The listing builds one solid part. Answer for the finished solid, in the listing's coordinates (mm). Face numbers are marked on the shaded views. A direction names the side the tool comes from. Give positions to 0.01 mm unless a question says otherwise; leave off trailing zeros. Loops run counter-clockwise (first coordinate to the right, second up) from the corner with the lowest first, then second, coordinate; pieces in that order, holes last. Notation, with made-up numbers: (-6, 56.25) - (6, 56.25) arc R20 cw to (6, 94.25) - close; hole circle Ø11 at (16, 21). An arc over 180 degrees is marked (long way). Write item = value, one per line. Start each with the question number.
1) Consider probe 1 along Z at (x, y) = (43.5, 22); probe 2 along Y at (x, z) = (63, 7.25); probe 3 along Y at (x, z) = (34.5, 4.25). Determine where each line is inside the solid, lowest interval first.
2) The part is cut by section C-C on z = 10.25. State how many separate pieces and enclosed holes the cut face has, plus the area to 3 significant figures.
3) Which of the six approach directions +Z, -Z, +X, -X, +Y, -Y give full straight-line access (tool end or side, diameter ignored) to the marked faces 1, 2, 3 and 4?
4) The part is cut by section B-B on x = 48.5. Write down the section's boundary in (y, z).
5) The mould has two halves that part along X. Classify the marked faces 5, 6 and 7: +X half, -X half, draft (parallel to the pull), parting line (faces both ways), or undercut.
6) Flat-ended cylindrical pins translate along their axes: P1, Ø1.5, axis at x = 74, z = 9, coming from the +Y side; P2, Ø7.5, axis at y = 44.5, z = 5, coming from the +X side; P3, Ø4.5, axis at y = 41, z = 6.5, coming from the +X side. Find the tip coordinate at first contact, or state that the pin passes through.
from build123d import *

# Parameters (mm, degrees)
BOSS_EXTRUDE1_DEPTH = 7
SKETCH1_3_R         = 7.578000113984699
BOSS_EXTRUDE2_DEPTH = 14.5
FILLET1_R           = 2


with BuildPart() as part:
    # Sketch1 → Boss-Extrude1 (new body)
    with BuildSketch(Plane.XY):
        with BuildLine():
            Line((78.96827475522947, 42.187825253742076), (71.54074542683735, 53.865587102003296))
            add(Edge.make_bspline(
                [(68.3903409242589, 57.6204965379541), (68.60270993607134, 57.450222077167965), (69.77589066925935, 56.287697416771124), (70.76711290567236, 54.99803586851411), (71.54074542683735, 53.865587102003296)],
                knots=[0.22419046507503326, 0.22419046507503326, 0.22419046507503326, 0.22419046507503326, 0.35338295041403034, 1, 1, 1, 1], degree=3))
            add(Edge.make_bspline(
                [(67.16681294608784, 58.3330475317527), (67.53066578937491, 58.14815845494029), (67.96561960838265, 57.94613577996738), (68.34100319904479, 57.66005482607508), (68.3903409242589, 57.6204965379541)],
                knots=[0, 0, 0, 0, 0.19417637174294056, 0.22419046507503326, 0.22419046507503326, 0.22419046507503326, 0.22419046507503326], degree=3))
            Line((67.16681294608784, 58.3330475317527), (56.03811631838445, 62.90331689854259))
            Line((56.03811631838445, 62.90331689854259), (50.21233359803197, 48.7174203330503))
            Line((50.21233359803197, 48.7174203330503), (52.95464713088683, 47.643030748312306))
            ThreePointArc((52.95464713088681, 47.64303074831224), (57.760447877225054, 40.24223776631537), (52.30143900683574, 33.30922401118043))
            Line((52.30143900683574, 33.30922401118043), (20.622854324708115, 24.120186594388674))
            Line((20.622854324708115, 24.120186594388674), (20.62282110130341, 6.139939904360626))
            Line((20.62282110130341, 6.139939904360626), (20.62282110130341, 6.062388021954931))
            Line((20.62282110130341, 6.062388021954931), (83.96827475522947, 15.843555634253288))
            add(Edge.make_bspline(
                [(83.96827475522947, 15.843555634253288), (85.80036579939097, 15.861062531667944), (88.17372578299519, 16.28932128394429), (90.97579799916589, 17.070964386264627), (92.71201966041953, 17.824393939393527), (94.43214299682957, 19.052982353729515), (96.04268050119445, 20.454120961956406), (97.16419489006465, 21.752212782610812), (97.85208586964548, 22.923017737887626), (98.59154777476378, 23.895634779714683), (99.07674499256737, 25.078186890956406), (99.65372100416238, 26.703400446360803), (99.9224179321126, 28.680656555027426), (100.1456525457167, 30.848800013363814), (100.51886620718611, 32.862374788732254), (101.11013591134653, 34.64525635165334), (101.50715414680975, 36.22789720071845), (102.06593723414899, 37.400646367775394), (102.48628027717764, 38.406589288866975), (102.84842112165893, 39.429390424414976), (103.21090056683431, 39.99039765339784), (103.38837792674808, 40.31628873971178)],
                knots=[0, 0, 0, 0, 0.1578550410840074, 0.20703944686554082, 0.2510949501731389, 0.3205511449351055, 0.3885120157665865, 0.43536001171879174, 0.4678008080744776, 0.5056992154510483, 0.5402779798217185, 0.5775724755717133, 0.6545316786338135, 0.7114166705153907, 0.7661367857027547, 0.8308692773593267, 0.873613048584834, 0.90658473443976, 0.9427498705208139, 0.9678813230428206, 1, 1, 1, 1], degree=3))
            Line((103.38837792674808, 40.31628873971178), (103.5353457354515, 40.58470837115218))
            Line((103.5353457354515, 40.58470837115218), (98.46827475522947, 40.584708371152175))
            Line((98.46827475522947, 40.584708371152175), (98.46827475522947, 57.7986883791206))
            Line((98.46827475522947, 57.7986883791206), (88.96827475522947, 57.7986883791206))
            Line((88.96827475522947, 57.7986883791206), (88.96827475522946, 31.5935556342533))
            ThreePointArc((88.96827475522946, 31.5935556342533), (83.96827475522947, 26.593555634253313), (78.96827475522949, 31.593555634253303))
            Line((78.96827475522947, 31.593555634253303), (78.96827475522947, 42.187825253742076))
        make_face()
    extrude(amount=BOSS_EXTRUDE1_DEPTH)

    # Sketch1_3 → Boss-Extrude2 (add)
    with BuildSketch(Plane.XY):
        with BuildLine():
            Line((52.95464713088683, 47.643030748312306), (50.21233359803197, 48.7174203330503))
            Line((50.21233359803197, 48.7174203330503), (23.91329061275728, 59.02091682731907))
            Line((23.91329061275728, 59.02091682731907), (22.08936487086497, 54.365458215317176))
            Line((22.08936487086497, 54.365458215317176), (40.01978708427513, 47.34063824296787))
            Line((40.01978708427513, 47.34063824296787), (44.49575262392416, 45.58703468895018))
            ThreePointArc((44.49575262392417, 45.58703468895018), (48.4005247200828, 47.95082949329833), (52.95464713088681, 47.64303074831224))
        make_face()
        with Locations((50.19030425910602, 40.58721795212874)):
            Circle(SKETCH1_3_R)
        with BuildLine():
            ThreePointArc((43.63005434703988, 36.79390715299979), (42.648765078906784, 41.32969523869845), (44.49575262392417, 45.58703468895018))
            Line((44.49575262392416, 45.58703468895018), (40.01978708427513, 47.34063824296787))
            Line((40.01978708427513, 47.34063824296787), (40.019787084275116, 35.746673468318164))
            Line((40.01978708427511, 35.74667346831816), (43.63005434703988, 36.79390715299979))
        make_face()
        with BuildLine():
            Line((20.622854324708115, 24.120186594388674), (52.30143900683574, 33.30922401118043))
            ThreePointArc((52.30143900683574, 33.30922401118043), (47.364634323302816, 33.55574050130448), (43.63005434703988, 36.79390715299979))
            Line((43.63005434703988, 36.79390715299979), (40.01978708427511, 35.74667346831816))
            Line((40.01978708427511, 35.74667346831816), (20.622854324708136, 30.12018659438867))
            Line((20.622854324708136, 30.12018659438867), (20.622854324708115, 24.120186594388674))
        make_face()
        with BuildLine():
            Line((108.09825459829777, 40.58470837115217), (103.53534573545149, 40.58470837115218))
            Line((103.5353457354515, 40.58470837115218), (103.38837792674808, 40.31628873971178))
            add(Edge.make_bspline(
                [(83.96827475522947, 15.843555634253288), (85.80036579939097, 15.861062531667944), (88.17372578299519, 16.28932128394429), (90.97579799916589, 17.070964386264627), (92.71201966041953, 17.824393939393527), (94.43214299682957, 19.052982353729515), (96.04268050119445, 20.454120961956406), (97.16419489006465, 21.752212782610812), (97.85208586964548, 22.923017737887626), (98.59154777476378, 23.895634779714683), (99.07674499256737, 25.078186890956406), (99.65372100416238, 26.703400446360803), (99.9224179321126, 28.680656555027426), (100.1456525457167, 30.848800013363814), (100.51886620718611, 32.862374788732254), (101.11013591134653, 34.64525635165334), (101.50715414680975, 36.22789720071845), (102.06593723414899, 37.400646367775394), (102.48628027717764, 38.406589288866975), (102.84842112165893, 39.429390424414976), (103.21090056683431, 39.99039765339784), (103.38837792674808, 40.31628873971178)],
                knots=[0, 0, 0, 0, 0.1578550410840074, 0.20703944686554082, 0.2510949501731389, 0.3205511449351055, 0.3885120157665865, 0.43536001171879174, 0.4678008080744776, 0.5056992154510483, 0.5402779798217185, 0.5775724755717133, 0.6545316786338135, 0.7114166705153907, 0.7661367857027547, 0.8308692773593267, 0.873613048584834, 0.90658473443976, 0.9427498705208139, 0.9678813230428206, 1, 1, 1, 1], degree=3))
            Line((83.96827475522947, 15.843555634253288), (40.01978708427512, 9.057472349332496))
            Line((40.01978708427512, 9.057472349332496), (20.62282110130341, 6.062388021954931))
            Line((20.62282110130341, 6.062388021954931), (20.62282110130341, 1.512651604953091))
            Line((20.6228211013034, 1.512651604953092), (99.05570161577305, 13.035195870356917))
            Line((99.05570161577305, 13.035195870356915), (108.09825459829777, 40.58470837115217))
        make_face()
        with BuildLine():
            Line((78.96827475522947, 42.187825253742076), (78.96827475522947, 43.59355563425329))
            Line((78.96827475522947, 43.59355563425329), (78.96827475522947, 49.285790380927594))
            Line((78.96827475522947, 49.285790380927594), (78.96827475522947, 52.81430633566804))
            Line((78.96827475522947, 52.81430633566804), (78.96827475522947, 53.14598079095306))
            Line((78.96827475522947, 53.14598079095306), (77.37761026058446, 54.95096484877639))
            Line((77.37761026058446, 54.95096484877639), (70.50082285395956, 62.75430218344684))
            Line((70.50082285395956, 62.75430218344684), (68.3903409242587, 57.62049653795411))
            add(Edge.make_bspline(
                [(68.3903409242589, 57.6204965379541), (68.60270993607134, 57.450222077167965), (69.77589066925935, 56.287697416771124), (70.76711290567236, 54.99803586851411), (71.54074542683735, 53.865587102003296)],
                knots=[0.22419046507503326, 0.22419046507503326, 0.22419046507503326, 0.22419046507503326, 0.35338295041403034, 1, 1, 1, 1], degree=3))
            Line((71.54074542683735, 53.865587102003296), (77.94135898527813, 43.80236991179886))
            Line((77.94135898527813, 43.80236991179886), (78.96827475522947, 42.187825253742076))
        make_face()
        with BuildLine():
            add(Edge.make_bspline(
                [(67.16681294608784, 58.3330475317527), (67.53066578937491, 58.14815845494029), (67.96561960838265, 57.94613577996738), (68.34100319904479, 57.66005482607508), (68.3903409242589, 57.6204965379541)],
                knots=[0, 0, 0, 0, 0.19417637174294056, 0.22419046507503326, 0.22419046507503326, 0.22419046507503326, 0.22419046507503326], degree=3))
            Line((68.3903409242587, 57.62049653795411), (70.50082285395956, 62.75430218344684))
            Line((70.50082285395956, 62.75430218344684), (57.93755222306168, 67.52848103011922))
            Line((57.93755222306168, 67.52848103011922), (56.03811631838445, 62.90331689854259))
            Line((56.03811631838445, 62.90331689854259), (67.16681294608784, 58.3330475317527))
        make_face()
    extrude(amount=BOSS_EXTRUDE2_DEPTH)

    # Fillet1
    fillet1_edges = [part.edges().sort_by_distance(p)[0] for p in [
        (78.96827475522947, 53.14598079095306, 7.25),
        (70.50082285395956, 62.75430218344684, 7.25),
        (99.05570161577305, 13.035195870356915, 7.25),
        (108.09825459829777, 40.58470837115217, 7.25),
        (98.46827475522947, 57.7986883791206, 3.5),
        (88.96827475522947, 57.7986883791206, 3.5),
        (57.93755222306168, 67.52848103011922, 7.25),
        (56.03811631838445, 62.90331689854259, 10.75),
        (78.96827475522947, 42.187825253742076, 10.75),
        (20.622821101303405, 1.5126516049530916, 7.25),
        (20.622854324708115, 24.120186594388674, 10.75),
        (20.622854324708136, 30.12018659438867, 7.25),
        (23.91329061275728, 59.02091682731907, 7.25),
        (22.08936487086497, 54.365458215317176, 7.25),
        (40.01978708427513, 47.34063824296787, 7.25),
        (40.01978708427511, 35.746673468318164, 7.25),
        (20.62282110130341, 6.062388021954931, 10.75),
    ]]
    fillet(fillet1_edges, radius=FILLET1_R)


solid = part.part
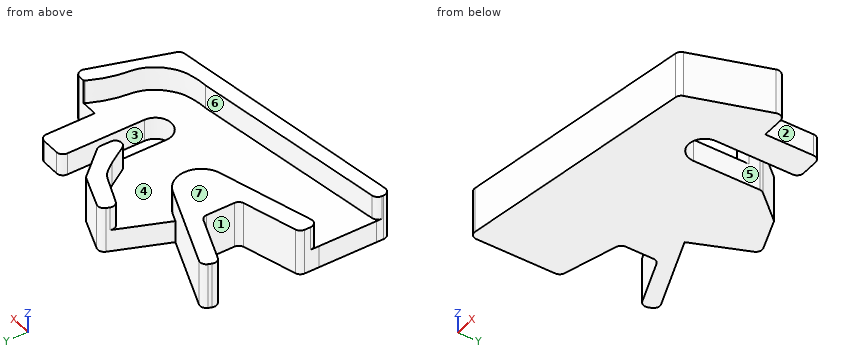
Answer below:
q1.probe_1 = 0 to 7
q1.probe_2 = 7.74 to 12.61, 60.04 to 65.6
q1.probe_3 = 3.55 to 34.15, 49.5 to 54.87
q2.separate_pieces = 3
q2.enclosed_holes = 0
q2.area = 1,130 mm2
q3.face_1 = +Z, -Z, -X
q3.face_2 = +Z, -Z, +X, +Y
q3.face_3 = +Z, -Z, +Y
q3.face_4 = +Z
q4.outline = (5.61, 0) - (49.39, 0) - (49.39, 14.5) - (32.21, 14.5) - (32.21, 7) - (10.37, 7) - (10.37, 14.5) - (5.61, 14.5) - close
q5.face_5 = undercut
q5.face_6 = -X half
q5.face_7 = draft
q6.P1 = 59.63
q6.P2 = 98.47
q6.P3 = 107.33
